CAD build for the part. Positions are in the model's coordinates, mm. A direction names the side the tool comes from. Coordinates: 2 decimals unless noted, no trailing zeros. Loops run counter-clockwise (first coordinate to the right, second up) from the corner with the lowest first, then second, coordinate; pieces in that order, holes last. Notation, with made-up numbers: (20, -35.5) -> (63, -35.5) arc R24 cw to (63, -25.5) -> close; hole circle Ø7 at (34.5, 83.25). An arc over 180 degrees is marked (long way). Answer as CSV lines item,"result". Start each with the question number.
from build123d import *

# Parameters (mm, degrees)
SKETCH1_R           = 29.35
BOSS_EXTRUDE1_DEPTH = 4
SKETCH1_4_R         = 6.55
SKETCH1_4_R_2       = 1.55
SKETCH1_4_R_3       = 9.55
CUT_EXTRUDE1_DEPTH  = 42.699460428
CUT_EXTRUDE2_START  = -1.5
SKETCH1_5_R         = 8.55
SKETCH1_5_R_2       = 6.55
CUT_EXTRUDE2_DEPTH  = 41.199460428
CUT_EXTRUDE3_START  = -2
SKETCH1_6_R         = 10.55
SKETCH1_6_R_2       = 9.55
CUT_EXTRUDE3_DEPTH  = 40.699460428
SKETCH1_7_R         = 3
SKETCH1_7_R_2       = 1.55
CUT_EXTRUDE4_DEPTH  = 3


with BuildPart() as part:
    # Sketch1 → Boss-Extrude1 (new body)
    with BuildSketch(Plane(origin=(0, 0, 0), x_dir=(1, 0, 0), z_dir=(0, 1, 0))):
        with Locations(Location((0, 0, 0), (0, 0, 270))):
            Circle(SKETCH1_R)
    extrude(amount=-BOSS_EXTRUDE1_DEPTH)

    # Sketch1_4 → Cut-Extrude1 (cut, through all)
    with BuildSketch(Plane(origin=(0, 0, 0), x_dir=(1, 0, 0), z_dir=(0, 1, 0))):
        with Locations(Location((-20, 0, 0), (0, 0, 270))):
            Circle(SKETCH1_4_R)
        with Locations(Location((-10, -17.320508076, 0), (0, 0, 270))):
            Circle(SKETCH1_4_R)
        with Locations(Location((10, -17.320508076, 0), (0, 0, 270))):
            Circle(SKETCH1_4_R)
        with Locations(Location((20, 0, 0), (0, 0, 270))):
            Circle(SKETCH1_4_R)
        with Locations(Location((10, 17.320508076, 0), (0, 0, 270))):
            Circle(SKETCH1_4_R)
        with Locations(Location((-10, 17.320508076, 0), (0, 0, 270))):
            Circle(SKETCH1_4_R)
        with Locations(Location((-21.650635095, -12.5, 0), (0, 0, 270))):
            Circle(SKETCH1_4_R_2)
        with Locations(Location((0, -25, 0), (0, 0, 270))):
            Circle(SKETCH1_4_R_2)
        with Locations(Location((21.650635095, -12.5, 0), (0, 0, 270))):
            Circle(SKETCH1_4_R_2)
        with Locations(Location((21.650635095, 12.5, 0), (0, 0, 270))):
            Circle(SKETCH1_4_R_2)
        with Locations(Location((0, 25, 0), (0, 0, 270))):
            Circle(SKETCH1_4_R_2)
        with Locations(Location((-21.650635095, 12.5, 0), (0, 0, 270))):
            Circle(SKETCH1_4_R_2)
        with Locations(Location((0, 0, 0), (0, 0, 270))):
            Circle(SKETCH1_4_R_3)
    extrude(amount=-CUT_EXTRUDE1_DEPTH, mode=Mode.SUBTRACT)

    # Sketch1_5 → Cut-Extrude2 (cut, through all)
    # profile 1 of 6: a face of its own
    with BuildSketch(Plane(origin=(0, 0, 0), x_dir=(1, 0, 0), z_dir=(0, 1, 0)).offset(CUT_EXTRUDE2_START)):
        with Locations(Location((-20, 0, 0), (0, 0, 270))):
            Circle(SKETCH1_5_R)
        with Locations(Location((-20, 0, 0), (0, 0, 270))):
            Circle(SKETCH1_5_R_2, mode=Mode.SUBTRACT)
    # profile 2 of 6: a face of its own
    with BuildSketch(Plane(origin=(0, 0, 0), x_dir=(1, 0, 0), z_dir=(0, 1, 0)).offset(CUT_EXTRUDE2_START)):
        with Locations(Location((-10, 17.320508076, 0), (0, 0, 270))):
            Circle(SKETCH1_5_R)
        with Locations(Location((-10, 17.320508076, 0), (0, 0, 270))):
            Circle(SKETCH1_5_R_2, mode=Mode.SUBTRACT)
    # profile 3 of 6: a face of its own
    with BuildSketch(Plane(origin=(0, 0, 0), x_dir=(1, 0, 0), z_dir=(0, 1, 0)).offset(CUT_EXTRUDE2_START)):
        with Locations(Location((10, 17.320508076, 0), (0, 0, 270))):
            Circle(SKETCH1_5_R)
        with Locations(Location((10, 17.320508076, 0), (0, 0, 270))):
            Circle(SKETCH1_5_R_2, mode=Mode.SUBTRACT)
    # profile 4 of 6: a face of its own
    with BuildSketch(Plane(origin=(0, 0, 0), x_dir=(1, 0, 0), z_dir=(0, 1, 0)).offset(CUT_EXTRUDE2_START)):
        with Locations(Location((20, 0, 0), (0, 0, 270))):
            Circle(SKETCH1_5_R)
        with Locations(Location((20, 0, 0), (0, 0, 270))):
            Circle(SKETCH1_5_R_2, mode=Mode.SUBTRACT)
    # profile 5 of 6: a face of its own
    with BuildSketch(Plane(origin=(0, 0, 0), x_dir=(1, 0, 0), z_dir=(0, 1, 0)).offset(CUT_EXTRUDE2_START)):
        with Locations(Location((10, -17.320508076, 0), (0, 0, 270))):
            Circle(SKETCH1_5_R)
        with Locations(Location((10, -17.320508076, 0), (0, 0, 270))):
            Circle(SKETCH1_5_R_2, mode=Mode.SUBTRACT)
    # profile 6 of 6: a face of its own
    with BuildSketch(Plane(origin=(0, 0, 0), x_dir=(1, 0, 0), z_dir=(0, 1, 0)).offset(CUT_EXTRUDE2_START)):
        with Locations(Location((-10, -17.320508076, 0), (0, 0, 270))):
            Circle(SKETCH1_5_R)
        with Locations(Location((-10, -17.320508076, 0), (0, 0, 270))):
            Circle(SKETCH1_5_R_2, mode=Mode.SUBTRACT)
    extrude(amount=-CUT_EXTRUDE2_DEPTH, mode=Mode.SUBTRACT)

    # Sketch1_6 → Cut-Extrude3 (cut, through all)
    with BuildSketch(Plane(origin=(0, 0, 0), x_dir=(1, 0, 0), z_dir=(0, 1, 0)).offset(CUT_EXTRUDE3_START)):
        with Locations(Location((0, 0, 0), (0, 0, 270))):
            Circle(SKETCH1_6_R)
        with Locations(Location((0, 0, 0), (0, 0, 270))):
            Circle(SKETCH1_6_R_2, mode=Mode.SUBTRACT)
    extrude(amount=-CUT_EXTRUDE3_DEPTH, mode=Mode.SUBTRACT)

    # Sketch1_7 → Cut-Extrude4 (cut)
    # profile 1 of 6: a face of its own
    with BuildSketch(Plane(origin=(0, 0, 0), x_dir=(1, 0, 0), z_dir=(0, 1, 0))):
        with Locations(Location((-21.650635095, 12.5, 0), (0, 0, 270))):
            Circle(SKETCH1_7_R)
        with Locations(Location((-21.650635095, 12.5, 0), (0, 0, 270))):
            Circle(SKETCH1_7_R_2, mode=Mode.SUBTRACT)
    # profile 2 of 6: a face of its own
    with BuildSketch(Plane(origin=(0, 0, 0), x_dir=(1, 0, 0), z_dir=(0, 1, 0))):
        with Locations(Location((0, 25, 0), (0, 0, 270))):
            Circle(SKETCH1_7_R)
        with Locations(Location((0, 25, 0), (0, 0, 270))):
            Circle(SKETCH1_7_R_2, mode=Mode.SUBTRACT)
    # profile 3 of 6: a face of its own
    with BuildSketch(Plane(origin=(0, 0, 0), x_dir=(1, 0, 0), z_dir=(0, 1, 0))):
        with Locations(Location((21.650635095, 12.5, 0), (0, 0, 270))):
            Circle(SKETCH1_7_R)
        with Locations(Location((21.650635095, 12.5, 0), (0, 0, 270))):
            Circle(SKETCH1_7_R_2, mode=Mode.SUBTRACT)
    # profile 4 of 6: a face of its own
    with BuildSketch(Plane(origin=(0, 0, 0), x_dir=(1, 0, 0), z_dir=(0, 1, 0))):
        with Locations(Location((21.650635095, -12.5, 0), (0, 0, 270))):
            Circle(SKETCH1_7_R)
        with Locations(Location((21.650635095, -12.5, 0), (0, 0, 270))):
            Circle(SKETCH1_7_R_2, mode=Mode.SUBTRACT)
    # profile 5 of 6: a face of its own
    with BuildSketch(Plane(origin=(0, 0, 0), x_dir=(1, 0, 0), z_dir=(0, 1, 0))):
        with Locations(Location((0, -25, 0), (0, 0, 270))):
            Circle(SKETCH1_7_R)
        with Locations(Location((0, -25, 0), (0, 0, 270))):
            Circle(SKETCH1_7_R_2, mode=Mode.SUBTRACT)
    # profile 6 of 6: a face of its own
    with BuildSketch(Plane(origin=(0, 0, 0), x_dir=(1, 0, 0), z_dir=(0, 1, 0))):
        with Locations(Location((-21.650635095, -12.5, 0), (0, 0, 270))):
            Circle(SKETCH1_7_R)
        with Locations(Location((-21.650635095, -12.5, 0), (0, 0, 270))):
            Circle(SKETCH1_7_R_2, mode=Mode.SUBTRACT)
    extrude(amount=-CUT_EXTRUDE4_DEPTH, mode=Mode.SUBTRACT)


solid = part.part
Item 1: Which spindle directions (+Z, -Z, +X, -X, +Y, -Y) get a long thin tool onto all of the face, cutting with end or side? Do faces 1 (the face through (-1.3, -3, -23.7)), 2 (the face through (-15, -1.5, 22)), 3 (the face through (16.494, -0.74, -18.173)). Say none if no direction does.
Item 2: Two-plate mould, pull along Z, no slides. Class faces 4 (the face through (9, -4, 6)), 5 (the face through (-23, -3, 14)): pulls with the +Z half, pulls with the -Z half, needs draft (parallel to the pull), parting line crosses it, or undercut.
Item 3: Saw through at D-D (x = -7). Write the cut outline in (y, z), plus the area to 3 significant figures.
Item 4: Saw through at B-B (y = -0.6). Count the separate pieces of the cut face and the enclosed holes in it, plus the area to 3 significant figures.
Item 5: Saw through at A-A (x = 0). Write the cut outline in (y, z).
Item 6: Flat gauge pins, fed straight in: pin 1 Ø10.5 at (x, z) = (-1.5, 0.5) entering from -Y; pin 2 Ø5 at (x, z) = (23.5, 3) entering from -Y; pin 3 Ø1.5 at (x, y) = (10.5, -2) entering from +Z; pin 4 Ø3 at (x, z) = (21.5, 11.5) entering from +Y. Where does each tip first touch, or does it go through?
Item 7: Saw through at C-C (z = 25). Write the cut outline in (x, y), plus the area to 3 significant figures.
Item 8: Wall check: probe 1 along X at (y, z) = (-3.5, 0); probe 2 along X at (y, z) = (-0.9, 12.5); probe 3 along X at (y, z) = (-3.25, 12.5). Give the ranges that are in metal, low to high.
Geometry check:
1,face 1,"+Y"
1,face 2,"-Y"
1,face 3,"+Y, -Y"
2,face 4,"needs draft"
2,face 5,"undercut"
3,outline,"(-4, -28.5) -> (0, -28.5) -> (0, -23.14) -> (-1.5, -23.14) -> (-1.5, -25.33) -> (-4, -25.33) -> close; (-4, -9.31) -> (-1.5, -9.31) -> (-1.5, -11.5) -> (0, -11.5) -> (0, -6.5) -> (-2, -6.5) -> (-2, -7.89) -> (-4, -7.89) -> close; (-4, 7.89) -> (-2, 7.89) -> (-2, 6.5) -> (0, 6.5) -> (0, 11.5) -> (-1.5, 11.5) -> (-1.5, 9.31) -> (-4, 9.31) -> close; (-4, 25.33) -> (-1.5, 25.33) -> (-1.5, 23.14) -> (0, 23.14) -> (0, 28.5) -> (-4, 28.5) -> close"
3,area,"55.5 mm2"
4,separate pieces,"1"
4,enclosed holes,"13"
4,area,"1,440 mm2"
5,outline,"(-4, -29.35) -> (0, -29.35) -> (0, -28) -> (-3, -28) -> (-3, -26.55) -> (-4, -26.55) -> close; (-4, -23.45) -> (-3, -23.45) -> (-3, -22) -> (0, -22) -> (0, -9.55) -> (-2, -9.55) -> (-2, -10.55) -> (-4, -10.55) -> close; (-4, 10.55) -> (-2, 10.55) -> (-2, 9.55) -> (0, 9.55) -> (0, 22) -> (-3, 22) -> (-3, 23.45) -> (-4, 23.45) -> close; (-4, 26.55) -> (-3, 26.55) -> (-3, 28) -> (0, 28) -> (0, 29.35) -> (-4, 29.35) -> close"
6,pin 1,"through"
6,pin 2,"y = -1.5"
6,pin 3,"z = 27.68"
6,pin 4,"y = -3"
7,outline,"(-15.38, -4) -> (-13.76, -4) -> (-13.76, -1.5) -> (-6.24, -1.5) -> (-6.24, -4) -> (-1.55, -4) -> (-1.55, -3) -> (-3, -3) -> (-3, 0) -> (-15.38, 0) -> close; (1.55, -4) -> (6.24, -4) -> (6.24, -1.5) -> (13.76, -1.5) -> (13.76, -4) -> (15.38, -4) -> (15.38, 0) -> (3, 0) -> (3, -3) -> (1.55, -3) -> close"
7,area,"64.3 mm2"
8,probe 1,"-29.35 to -28.55, -11.45 to -10.55, 10.55 to 11.45, 28.55 to 29.35"
8,probe 2,"-26.56 to -24.65, -18.65 to -14.43, -5.57 to 5.57, 14.43 to 18.65, 24.65 to 26.56"
8,probe 3,"-26.56 to -23.2, -20.1 to -17.06, -2.94 to 2.94, 17.06 to 20.1, 23.2 to 26.56"
